```python
from build123d import *

# Parameters (mm, degrees)
F1_DEPTH       = 370
F2_R           = 4
F3_R           = 4
F5_D           = 8
F5_CSINK_D     = 10
F5_CSINK_ANGLE = 90
F7_D           = 9
F7_CSINK_D     = 10
F7_CSINK_ANGLE = 90


with BuildPart() as f1:
    # F0 (on Front) → F1 (new body)
    with BuildSketch(Plane.XZ):
        Polygon((38, 0), (0, 0), (0, -38), (6.3, -38), (6.3, -6.3), (38, -6.3), align=None)
    extrude(amount=F1_DEPTH)

    # F2
    f2_edges = [f1.edges().sort_by_distance(p)[0] for p in [
        (6.3, -185, -38),
        (38, -185, -6.3),
    ]]
    fillet(f2_edges, radius=F2_R)

    # F3
    f3_edges = [f1.edges().sort_by_distance(p)[0] for p in [
        (6.3, -185, -6.3),
    ]]
    fillet(f3_edges, radius=F3_R)

    # F5 (through all)
    with Locations(Plane.XY):
        with Locations((30, -341), (30, -237), (30, -133), (30, -29)):
            CounterSinkHole(F5_D / 2, F5_CSINK_D / 2, counter_sink_angle=F5_CSINK_ANGLE)

    # F7 (through all)
    with Locations(Plane(origin=(0, 0, 0), x_dir=(0, -1, 0), z_dir=(-1, 0, 0))):
        with Locations((310, -24), (60, -24.86)):
            CounterSinkHole(F7_D / 2, F7_CSINK_D / 2, counter_sink_angle=F7_CSINK_ANGLE)


solid = f1.part
```
CAD build for the part. Positions are in the model's coordinates, mm. A direction names the side the tool comes from. Coordinates: 2 decimals unless noted, no trailing zeros. Loops run counter-clockwise (first coordinate to the right, second up) from the corner with the lowest first, then second, coordinate; pieces in that order, holes last. Notation, with made-up numbers: (-36.5, 55.25) - (-15.5, 55.25) arc R14 cw to (-15.5, 80.25) - close; hole circle Ø7 at (56.25, -17). An arc over 180 degrees is marked (long way). Return JSON: item names as keys, results as strings.
1. Band-saw the part on C-C (z = -15). Give the cut face in (x, y), and give its area (3 significant figures).
Result:
{"outline": "(0, -370) - (6.3, -370) - (6.3, 0) - (0, 0) - close", "area": "2,330 mm2"}
2. 3-axis set-ups, long thin cutter, end or side, ignore diameter. For faces 1 (the flat face through (22, -182, -6.3)), 2 (the cylindrical face through (30.521, -129.034, -3.687)): which of +Z, -Z, +X, -X, +Y, -Y reach the whole face in a straight line?
Result:
{"face 1": "-Z, +X, +Y, -Y", "face 2": "+Z, -Z"}
3. Mould opens along X. For faces 3 (the flat face through (0, -182, -19)), 4 (the flat face through (6, 0, -10)), 5 (the cylindrical face through (28.154, -344.549, -3.687)), 6 (the cylindrical face through (30.521, -25.034, -3.687)) say: released by +X, released by -X, zero draft, split by the parting line, or undercut.
Result:
{"face 3": "released by -X", "face 4": "zero draft", "face 5": "undercut", "face 6": "undercut"}
4. Probe L1, parallel to Y at x = 30, z = -2; L2, parallel to Z at x = 17.5, y = -338.5; L3, parallel to X at y = -157.5, z = -25. List the from-to ranges inside material, lowest first. Write a range as from..to.
Result:
{"L1": "y = -370..-345, -337..-241, -233..-137, -129..-33, -25..0", "L2": "z = -6.3..0", "L3": "x = 0..6.3"}
5. Drop flat-ended pins along their axis: pin 1 (7 mm diameter, centred on x = 30, y = -237, fed in from -Z); pin 2 (8 mm diameter, centred on y = -248, z = -10, fed in from +X); pin 3 (7 mm diameter, centred on y = -264.5, z = -25.5, fed in from +X). Give the stop position or say it passes through.
Result:
{"pin 1": "passes through", "pin 2": "stops at x = 35.52", "pin 3": "stops at x = 6.3"}
6. Band-saw the part on A-A (y = -60). Give the cut face in (x, z), and give its area (3 significant figures).
Result:
{"outline": "(0, -38) - (2.3, -38) arc R4 ccw to (6.3, -34) - (6.3, -29.36) - (0.5, -29.36) - (0, -29.86) - close; (0, -19.86) - (0.5, -20.36) - (6.3, -20.36) - (6.3, -10.3) arc R4 cw to (10.3, -6.3) - (34, -6.3) arc R4 ccw to (38, -2.3) - (38, 0) - (0, 0) - close", "area": "379 mm2"}
7. Band-saw the part on B-B (x = 18). Give the cut face in (y, z), and give its area (3 significant figures).
Result:
{"outline": "(-370, -6.3) - (0, -6.3) - (0, 0) - (-370, 0) - close", "area": "2,330 mm2"}
